Input: part model. Units: mm. Frame: model coordinates. Face numbers are marked on the shaded views. A direction names the side the tool comes from. Round coordinates to 2 decimals unless told otherwise and drop trailing zeros. Order: outer loops, then holes, each group sorted by start corner. A loop starts at its lowest first (then second) coordinate and runs counter-clockwise, first axis right, second up. Notation, with made-up numbers: (62, 40) -> (108, 40) arc R27 cw to (108, 77) -> close; hole circle Ø1 at (31, -23). An arc over 180 degrees is marked (long way). Answer as CSV lines item,"result". Start each with the question number.
1) Line query: L1, parallel to X at y = 1.55, z = 0; L2, parallel to X at y = 1.5, z = -6.5; L3, parallel to Z at x = 0, y = 2.15. Output: solid intervals per line, ascending.
2) Section query C-C, the plane y = 18.25. Output: boundary loops of the cut face in (x, z) (3 decimals).
3) Section query A-A, the plane x = 0. Output: boundary loops of the cut face in (y, z), and give its area (3 significant figures).
4) Access query for the marked faces 4, 5, 6, 7 and 8. Directions: +Z, -Z, +X, -X, +Y, -Y. A direction counts if a zero-diameter tool reaches every point of the face in a straight line with its end or side. Return the directions, or none.
5) First-contact query: P1, Ø2, axis at y = 7.5, z = -17.5, coming from the -X side; P2, Ø1, axis at y = 18, z = -3.5, coming from the +X side; P3, Ø2, axis at x = 3.5, y = 8, coming from the -Z side; P4, Ø2, axis at x = -12.5, z = -20.5, coming from the -Y side. Flat tips, straight axial feed; report the tip coordinate or a pass-through.
6) Section query B-B, the plane y = 23.5. Output: boundary loops of the cut face in (x, z), and give its area (3 significant figures).
7) Mould query, pull axis Z, two halves, no side actions, for the marked faces 1, 2 and 3. Classes: +Z half, -Z half, draft (parallel to the pull), parting line (faces both ways), or undercut.
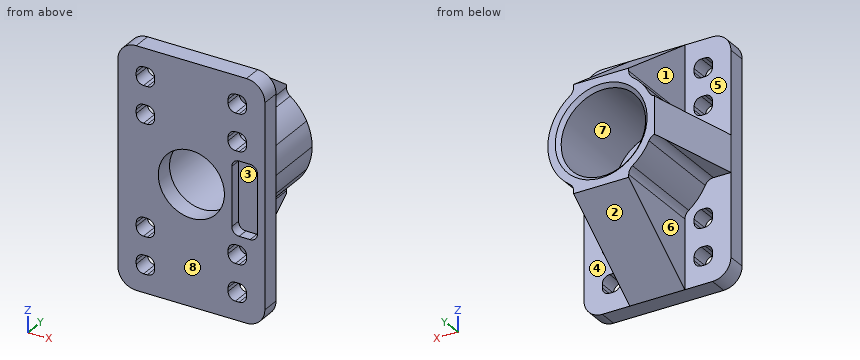
```python
from build123d import *

# Parameters (mm, degrees)
SKETCH1_W                       = 40
SKETCH1_H                       = 65
SKETCH1_W_2                     = 5
SKETCH1_H_2                     = 5
MOUNTBASE_DEPTH                 = 5
SKETCH4_R                       = 11.5
PIPEBASE_DEPTH                  = 25
RIB3_REACH                      = 50.541
SKETCH6_WALL_W                  = 124.680290668
SKETCH6_WALL_H                  = 10
RIB5_REACH                      = 50.541
SKETCH7_WALL_W                  = 129.888282796
SKETCH7_WALL_H                  = 15
BASEFILLET_R                    = 5
PIPEFILLET_R                    = 2.5
INNERMATERIALREMOVAL_DEPTH      = 46.620718977
INNERMATERIALREMOVAL_DEPTH_BACK = 46.620718977
SKETCH8_R                       = 9
PIPECHAMFER_SIZE                = 1
FILLET5_R                       = 2
CUT_EXTRUDE2_START              = -25
CUT_EXTRUDE2_DEPTH              = 25
SKETCH10_W                      = 7
SKETCH10_H                      = 20
CUT_EXTRUDE3_DEPTH              = 3
FILLET6_R                       = 2


with BuildPart() as part:
    # Sketch1 → MountBase (new body)
    with BuildSketch(Plane(origin=(0, 0, 0), x_dir=(1, 0, 0), z_dir=(0, 1, 0))):
        Rectangle(SKETCH1_W, SKETCH1_H)
        with Locations((-12.5, 15)):
            Rectangle(SKETCH1_W_2, SKETCH1_H_2, mode=Mode.SUBTRACT)
        with Locations((-12.5, -15)):
            Rectangle(SKETCH1_W_2, SKETCH1_H_2, mode=Mode.SUBTRACT)
        with Locations((12.5, 15)):
            Rectangle(SKETCH1_W_2, SKETCH1_H_2, mode=Mode.SUBTRACT)
        with Locations((12.5, -15)):
            Rectangle(SKETCH1_W_2, SKETCH1_H_2, mode=Mode.SUBTRACT)
        with Locations((-12.5, -25)):
            Rectangle(SKETCH1_W_2, SKETCH1_H_2, mode=Mode.SUBTRACT)
        with Locations((12.5, -25)):
            Rectangle(SKETCH1_W_2, SKETCH1_H_2, mode=Mode.SUBTRACT)
        with Locations((-12.5, 25)):
            Rectangle(SKETCH1_W_2, SKETCH1_H_2, mode=Mode.SUBTRACT)
        with Locations((12.5, 25)):
            Rectangle(SKETCH1_W_2, SKETCH1_H_2, mode=Mode.SUBTRACT)
    extrude(amount=MOUNTBASE_DEPTH)

    # Sketch4 → PipeBase (add)
    with BuildSketch(Plane(origin=(0, 5, 0), x_dir=(1, 0, 0), z_dir=(0, 1, 0))):
        with BuildLine():
            Line((-14.5, 5), (-14.5, -5))
            Line((-14.5, -5), (-13.610657589, -5))
            ThreePointArc((-13.610657589, -5), (-11.186634071, -9.225465742), (-7.5, -12.409673646))
            Line((-7.5, -12.409673646), (-7.5, -14.5))
            Line((-7.5, -14.5), (7.5, -14.5))
            Line((7.5, -14.5), (7.5, -12.409673646))
            ThreePointArc((7.5, -12.409673646), (11.186634071, -9.225465742), (13.610657589, -5))
            Line((13.610657589, -5), (14.5, -5))
            Line((14.5, -5), (14.5, 5))
            Line((14.5, 5), (13.610657589, 5))
            ThreePointArc((13.610657589, 5), (11.186634071, 9.225465742), (7.5, 12.409673646))
            Line((7.5, 12.409673646), (7.5, 14.5))
            Line((7.5, 14.5), (-7.5, 14.5))
            Line((-7.5, 14.5), (-7.5, 12.409673646))
            ThreePointArc((-7.5, 12.409673646), (-11.186634071, 9.225465742), (-13.610657589, 5))
            Line((-13.610657589, 5), (-14.5, 5))
        make_face()
        with Locations(Location((0, 0, 0), (0, 0, 270))):
            Circle(SKETCH4_R, mode=Mode.SUBTRACT)
    extrude(amount=PIPEBASE_DEPTH)

    # Sketch6 wall → Rib3 (add, up to next)
    with BuildSketch(Plane(origin=(-17.25, 17.5, 0), x_dir=(-0.214861782675, -0.976644466705, 0), z_dir=(0.976644466705, -0.214861782675, 0)), mode=Mode.PRIVATE) as rib3_sk1:
        Rectangle(SKETCH6_WALL_W, SKETCH6_WALL_H)
    rib3_tool1 = extrude(rib3_sk1.sketch, amount=RIB3_REACH, mode=Mode.PRIVATE) - part.part
    rib3 = rib3_tool1.solids().sort_by_distance((-17.25, 17.5, 0))[0]
    add(rib3)

    # Mirror1: Rib3 across plane
    add(rib3.mirror(Plane(origin=(0, 0, 0), x_dir=(0, 0, 1), z_dir=(1, 0, 0))))

    # Sketch7 wall → Rib5 (add, up to next)
    with BuildSketch(Plane(origin=(0, 17.5, 23.5), x_dir=(0, -0.811534341451, 0.584304725845), z_dir=(0, -0.584304725845, -0.811534341451)), mode=Mode.PRIVATE) as rib5_sk1:
        Rectangle(SKETCH7_WALL_W, SKETCH7_WALL_H)
    rib5_tool1 = extrude(rib5_sk1.sketch, amount=RIB5_REACH, mode=Mode.PRIVATE) - part.part
    rib5 = rib5_tool1.solids().sort_by_distance((0, 17.5, 23.5))[0]
    add(rib5)

    # Mirror2: Rib5 across plane
    add(rib5.mirror(Plane.XY))

    # BaseFillet
    basefillet_edges = [part.edges().sort_by_distance(p)[0] for p in [
        (20, 2.5, 32.5),
        (-20, 2.5, 32.5),
        (-20, 2.5, -32.5),
        (20, 2.5, -32.5),
    ]]
    fillet(basefillet_edges, radius=BASEFILLET_R)

    # PipeFillet
    # the kernel refuses this fillet: 2.5 mm, written as the material it adds along each edge
    with BuildSketch(Plane(origin=(-13.610657589, 0.886278216, -5), x_dir=(-1, 0, 0), z_dir=(0, 1, 0))) as pipefillet_piece_1_section:
        with BuildLine():
            CenterArc((1.645488714, -2.5), PIPEFILLET_R, 90, 63.821031296)
            ThreePointArc((-0.598062213, -1.397058824), (-0.280715993, -0.706369867), (0, 0))
            Line((0, 0), (1.645488714, 0))
        make_face()
    pipefillet_piece_1 = extrude(amount=29.113721784, mode=Mode.PRIVATE)
    pipefillet_piece_1 = split(pipefillet_piece_1, bisect_by=Plane(origin=(-20.148077302, 4.326921354, -5.304724049), z_dir=(0.976644466705111, -0.2148617826750244, 0)), keep=Keep.TOP, mode=Mode.PRIVATE)
    add(pipefillet_piece_1)
    with BuildSketch(Plane(origin=(-7.5, 1.654866403, -12.409673646), x_dir=(-0.8330213423374977, 0, 0.5532408546105696), z_dir=(0, 1, 0))) as pipefillet_piece_2:
        with BuildLine():
            CenterArc((1.342287528, -2.497729208), PIPEFILLET_R, 92.442244575, 53.968120928)
            Line((-0.740265828, -1.114627072), (0, 0))
            ThreePointArc((0, 0), (0.617878386, -0.013170592), (1.235756772, 0))
        make_face()
    extrude(amount=28.345133597)
    with BuildSketch(Plane(origin=(-13.610657589, 0.886278216, 5), x_dir=(-1, 0, 0), z_dir=(0, 1, 0))) as pipefillet_piece_3_section:
        with BuildLine():
            CenterArc((1.645488714, 2.5), PIPEFILLET_R, 206.178968704, 63.821031296)
            ThreePointArc((-0.598062213, 1.397058824), (-0.280715993, 0.706369867), (0, 0))
            Line((0, 0), (1.645488714, 0))
        make_face()
    pipefillet_piece_3 = extrude(amount=29.113721784, mode=Mode.PRIVATE)
    pipefillet_piece_3 = split(pipefillet_piece_3, bisect_by=Plane(origin=(-20.148077302, 4.326921354, 5.304724049), z_dir=(0.976644466705111, -0.2148617826750244, 0)), keep=Keep.TOP, mode=Mode.PRIVATE)
    add(pipefillet_piece_3)
    with BuildSketch(Plane(origin=(-7.5, 1.654866403, 12.409673646), x_dir=(-0.8330213423374981, 0, -0.5532408546105689), z_dir=(0, 1, 0))) as pipefillet_piece_4:
        with BuildLine():
            CenterArc((1.342287528, 2.497729208), PIPEFILLET_R, 213.589634497, 53.968120928)
            Line((-0.740265828, 1.114627072), (0, 0))
            ThreePointArc((0, 0), (0.617878386, 0.013170592), (1.235756772, 0))
        make_face()
    extrude(amount=28.345133597)
    with BuildSketch(Plane(origin=(7.5, 1.654866403, 12.409673646), x_dir=(0, 0, 1), z_dir=(0, 1, 0))) as pipefillet_piece_5:
        with BuildLine():
            CenterArc((1.338053439, 2.5), PIPEFILLET_R, 216.031879072, 53.968120928)
            ThreePointArc((-0.683671132, 1.029411765), (-0.330864182, 0.521992392), (0, 0))
            Line((0, 0), (1.338053439, 0))
        make_face()
    extrude(amount=28.345133597)
    with BuildSketch(Plane(origin=(13.610657589, 0.886278216, 5), x_dir=(1, 0, 0), z_dir=(0, 1, 0))) as pipefillet_piece_6_section:
        with BuildLine():
            CenterArc((1.645488714, -2.5), PIPEFILLET_R, 90, 63.821031296)
            ThreePointArc((-0.598062213, -1.397058824), (-0.280715993, -0.706369867), (0, 0))
            Line((0, 0), (1.645488714, 0))
        make_face()
    pipefillet_piece_6 = extrude(amount=29.113721784, mode=Mode.PRIVATE)
    pipefillet_piece_6 = split(pipefillet_piece_6, bisect_by=Plane(origin=(20.148077302, 4.326921354, 5.304724049), z_dir=(-0.976644466705111, -0.21486178267502437, 0)), keep=Keep.TOP, mode=Mode.PRIVATE)
    add(pipefillet_piece_6)
    with BuildSketch(Plane(origin=(13.610657589, 0.886278216, -5), x_dir=(-0.3935427494511154, 0, -0.9193063169338371), z_dir=(0, 1, 0))) as pipefillet_piece_7_section:
        with BuildLine():
            CenterArc((1.65069564, -2.496565042), PIPEFILLET_R, 93.003848679, 63.821031296)
            Line((-0.647570153, -1.512708169), (0, 0))
            ThreePointArc((0, 0), (0.759844025, -0.019922754), (1.519688049, 0))
        make_face()
    pipefillet_piece_7 = extrude(amount=29.113721784, mode=Mode.PRIVATE)
    pipefillet_piece_7 = split(pipefillet_piece_7, bisect_by=Plane(origin=(20.148077302, 4.326921354, -5.304724049), z_dir=(-0.976644466705111, -0.21486178267502437, 0)), keep=Keep.TOP, mode=Mode.PRIVATE)
    add(pipefillet_piece_7)
    with BuildSketch(Plane(origin=(7.5, 1.654866403, -12.409673646), x_dir=(0, 0, -1), z_dir=(0, 1, 0))) as pipefillet_piece_8:
        with BuildLine():
            CenterArc((1.338053439, -2.5), PIPEFILLET_R, 90, 53.968120928)
            ThreePointArc((-0.683671132, -1.029411765), (-0.330864182, -0.521992392), (0, 0))
            Line((0, 0), (1.338053439, 0))
        make_face()
    extrude(amount=28.345133597)

    # Sketch8 → InnerMaterialRemoval (cut, two sides: drawn at the far end of the back side and taken through both)
    with BuildSketch(Plane(origin=(0, 5, 0), x_dir=(1, 0, 0), z_dir=(0, 1, 0)).offset(-INNERMATERIALREMOVAL_DEPTH_BACK)):
        with Locations(Location((0, 0, 0), (0, 0, 270))):
            Circle(SKETCH8_R)
    extrude(amount=INNERMATERIALREMOVAL_DEPTH + INNERMATERIALREMOVAL_DEPTH_BACK, mode=Mode.SUBTRACT)

    # PipeChamfer
    pipechamfer_edges = [part.edges().sort_by_distance(p)[0] for p in [
        (0, 30, -11.5),
    ]]
    chamfer(pipechamfer_edges, length=PIPECHAMFER_SIZE)

    # Fillet5
    fillet5_edges = [part.edges().sort_by_distance(p)[0] for p in [
        (10, 2.5, -27.5),
        (10, 2.5, -22.5),
        (15, 2.5, -22.5),
        (15, 2.5, -27.5),
        (-10, 2.5, -12.5),
        (-10, 2.5, -17.5),
        (-15, 2.5, -17.5),
        (-15, 2.5, -12.5),
        (-10, 2.5, 17.5),
        (-10, 2.5, 12.5),
        (-15, 2.5, 12.5),
        (-15, 2.5, 17.5),
        (15, 2.5, -12.5),
        (15, 2.5, -17.5),
        (10, 2.5, -17.5),
        (10, 2.5, -12.5),
        (15, 2.5, 17.5),
        (15, 2.5, 12.5),
        (10, 2.5, 12.5),
        (10, 2.5, 17.5),
        (-10, 2.5, 27.5),
        (-10, 2.5, 22.5),
        (-15, 2.5, 22.5),
        (-15, 2.5, 27.5),
        (15, 2.5, 27.5),
        (15, 2.5, 22.5),
        (10, 2.5, 22.5),
        (10, 2.5, 27.5),
        (-15, 2.5, -27.5),
        (-15, 2.5, -22.5),
        (-10, 2.5, -22.5),
        (-10, 2.5, -27.5),
    ]]
    fillet(fillet5_edges, radius=FILLET5_R)

    # Sketch9 → Cut-Extrude2 (cut)
    with BuildSketch(Plane(origin=(0, 30, 0), x_dir=(1, 0, 0), z_dir=(0, 1, 0)).offset(CUT_EXTRUDE2_START)):
        with BuildLine():
            Line((7.5, -13.747727085), (8.27770049, -13.747727085))
            Line((8.27770049, -13.747727085), (20, -7.665046243))
            Line((20, -7.665046243), (20, 7.665046243))
            Line((20, 7.665046243), (8.27770049, 13.747727085))
            Line((8.27770049, 13.747727085), (7.5, 13.747727085))
            ThreePointArc((7.5, 13.747727085), (7.772168028, 12.613370569), (8.529411765, 11.726002514))
            ThreePointArc((8.529411765, 11.726002514), (11.095671594, 9.334670422), (13.012595376, 6.397058824))
            ThreePointArc((13.012595376, 6.397058824), (13.625464362, 5.605039206), (14.5, 5.11709363))
            Line((14.5, 5.11709363), (14.5, -5.11709363))
            ThreePointArc((14.5, -5.11709363), (13.625464362, -5.605039206), (13.012595376, -6.397058824))
            ThreePointArc((13.012595376, -6.397058824), (11.095671594, -9.334670422), (8.529411765, -11.726002514))
            ThreePointArc((8.529411765, -11.726002514), (7.772168028, -12.613370569), (7.5, -13.747727085))
        make_face()
        with BuildLine():
            ThreePointArc((14.5, 5.11709363), (13.625464362, 5.605039206), (13.012595376, 6.397058824))
            ThreePointArc((13.012595376, 6.397058824), (14.123254458, 3.283851934), (14.5, 0))
            Line((14.5, 0), (14.5, 5.11709363))
        make_face()
        with BuildLine():
            Line((14.5, -5.11709363), (14.5, 0))
            ThreePointArc((14.5, 0), (14.123254458, -3.283851934), (13.012595376, -6.397058824))
            ThreePointArc((13.012595376, -6.397058824), (13.625464362, -5.605039206), (14.5, -5.11709363))
        make_face()
    extrude(amount=CUT_EXTRUDE2_DEPTH, mode=Mode.SUBTRACT)

    # Sketch10 → Cut-Extrude3 (cut)
    with BuildSketch(Plane.XZ):
        with Locations((14.5, 0)):
            Rectangle(SKETCH10_W, SKETCH10_H)
    extrude(amount=-CUT_EXTRUDE3_DEPTH, mode=Mode.SUBTRACT)

    # Fillet6
    fillet6_edges = [part.edges().sort_by_distance(p)[0] for p in [
        (18, 1.5, 10),
        (18, 1.5, -10),
        (11, 1.5, -10),
        (11, 1.5, 10),
    ]]
    fillet(fillet6_edges, radius=FILLET6_R)


solid = part.part
```
Findings:
1,L1,"x = -20 to -9, 9 to 11, 18 to 20"
1,L2,"x = -20 to -6.22, 6.22 to 11, 18 to 20"
1,L3,"z = -32.5 to -9, 9 to 32.5"
2,outline,"(-17.085, -5) -> (-15.256, -5) arc R2.5 cw to (-13.013, -6.397) arc R14.5 ccw to (-8.529, -11.726) arc R2.5 cw to (-7.5, -13.748) -> (-7.5, -22.96) -> (7.5, -22.96) -> (7.5, -13.748) arc R2.5 cw to (8.529, -11.726) arc R14.5 ccw to (8.529, 11.726) arc R2.5 cw to (7.5, 13.748) -> (7.5, 22.96) -> (-7.5, 22.96) -> (-7.5, 13.748) arc R2.5 cw to (-8.529, 11.726) arc R14.5 ccw to (-13.013, 6.397) arc R2.5 cw to (-15.256, 5) -> (-17.085, 5) -> close; hole circle Ø23 at (0, 0)"
3,outline,"(0, -32.5) -> (5, -32.5) -> (30, -14.5) -> (30, -12.5) -> (29, -11.5) -> (5, -11.5) -> (5, -9) -> (0, -9) -> close; (0, 9) -> (5, 9) -> (5, 11.5) -> (29, 11.5) -> (30, 12.5) -> (30, 14.5) -> (5, 32.5) -> (0, 32.5) -> close"
3,area,"834 mm^2"
4,face 4,"+X, +Y"
4,face 5,"+Z, -X, +Y"
4,face 6,"-Z, -X, +Y"
4,face 7,"+Y"
4,face 8,"+Z, -Z, +X, -X, -Y"
5,P1,"stops at x = -7.5"
5,P2,"stops at x = 14.19"
5,P3,"stops at z = -31.06"
5,P4,"stops at y = 0"
6,outline,"(-15.93, -5) -> (-15.26, -5) arc R2.5 cw to (-13.01, -6.4) arc R14.5 ccw to (-8.53, -11.73) arc R2.5 cw to (-7.5, -13.75) -> (-7.5, -19.18) -> (7.5, -19.18) -> (7.5, -13.75) arc R2.5 cw to (8.53, -11.73) arc R14.5 ccw to (8.53, 11.73) arc R2.5 cw to (7.5, 13.75) -> (7.5, 19.18) -> (-7.5, 19.18) -> (-7.5, 13.75) arc R2.5 cw to (-8.53, 11.73) arc R14.5 ccw to (-13.01, 6.4) arc R2.5 cw to (-15.26, 5) -> (-15.93, 5) -> close; hole circle Ø23 at (0, 0)"
6,area,"425 mm^2"
7,face 1,"draft"
7,face 2,"-Z half"
7,face 3,"undercut"
